Work out the finished part from the listing and answer in its coordinate system (mm). A direction names the side the tool comes from. Give positions to 0.01 mm unless a question says otherwise; leave off trailing zeros. Loops run counter-clockwise (first coordinate to the right, second up) from the corner with the lowest first, then second, coordinate; pieces in that order, holes last.
Autodesk Inventor part; units mm, degrees
ref_plane "YZ Plane" through (0, 0, 0) normal (1, 0, 0) x (0, 1, 0)
ref_plane "XZ Plane" through (0, 0, 0) normal (0, 1, 0) x (-1, 0, 0)
ref_plane "XY Plane" through (0, 0, 0) normal (0, 0, 1) x (1, 0, 0)
sketch "Sketch1" plane through (0, 0, 0) normal (0, 0, 1) x (1, 0, 0)
  circle A0 centre (0, 0) radius 59
  circle A1 centre (90, 0) radius 59
  line L0 (0, 59) -> (90, 59)
  line L1 (90, -59) -> (0, -59)
  dimension "d0" = 118
  dimension "d1" = 118
  dimension "d2" = 90
extrude "Extrusion1" add sketch "Sketch1" along normal blind 5
sketch "Sketch2" plane through (0, 0, 0) normal (0, 0, -1) x (-1, 0, 0)
  arc A0 (0, -59) -> (0, 59) centre (0, 0) ccw
  line L0 (-90, 59) -> (0, 59)
  arc A1 (-90, 59) -> (-90, -59) centre (-90, 0) ccw
  line L1 (0, -59) -> (-90, -59)
  arc A2 (0, -56) -> (0, 56) centre (0, 0) ccw
  line L2 (0, -56) -> (-90, -56)
  arc A3 (-90, 56) -> (-90, -56) centre (-90, 0) ccw
  line L3 (-90, 56) -> (0, 56)
  dimension "d5" = 3
extrude "Extrusion2" cut sketch "Sketch2" against normal blind 4 contours L2 A3 L3 A2
sketch "Sketch3" plane through (0, 0, 5) normal (0, 0, 1) x (1, 0, 0)
  circle A0 centre (90, 0) radius 7.5
  arc A1 (90, -59) -> (90, 59) centre (90, 0) ccw
  circle A2 centre (0, 0) radius 50
  dimension "d8" = 15
  dimension "d9" = 100
extrude "Extrusion3" cut sketch "Sketch3" against normal through all
sketch "Sketch4" plane through (0, 0, 5) normal (0, 0, 1) x (1, 0, 0)
  line L0 (45, 52.5) -> (45, -52.5) construction
  line L1 (90, 59) -> (0, 59) construction
  circle A0 centre (45, 52.5) radius 1.5
  circle A1 centre (45, -52.5) radius 1.5
  point P0 (0, 0)
  point P1 (45, 0)
  point P2 (45, 59)
  dimension "d12" = 105
  dimension "d13" = 3
  dimension "d14" = 3
extrude "Extrusion4" cut sketch "Sketch4" against normal through all
sketch "Sketch5" plane through (0, 0, 4) normal (0, 0, -1) x (-1, 0, 0)
  circle A0 centre (-45, -52.5) radius 1.5
  circle A1 centre (-45, 52.5) radius 1.5
  circle A2 centre (-45, 52.5) radius 6.5
  line L0 (-38.5, 52.5) -> (-38.5, 59)
  line L1 (-51.5, 52.5) -> (-51.5, 59)
  line L2 (-90, 59) -> (0, 59)
  line L3 (-38.5, 59) -> (-51.5, 59)
  line L4 (-51.5, 59) -> (-38.5, 59)
  circle A3 centre (-45, -52.5) radius 6.5
  line L5 (-38.5, -52.5) -> (-38.5, -59)
  line L6 (0, -59) -> (-90, -59)
  line L7 (-38.5, -59) -> (-51.5, -59)
  line L8 (-51.5, -59) -> (-51.5, -52.5)
  point P0 (0, 0)
  dimension "d17" = 13
  dimension "d18" = 13
extrude "Extrusion5" add sketch "Sketch5" along normal blind 4
sketch "Sketch6" plane through (0, 0, 5) normal (0, 0, 1) x (1, 0, 0)
  circle A0 centre (45, -52.5) radius 1.5
  circle A1 centre (45, 52.5) radius 1.5
  circle A2 centre (45, 52.5) radius 1.5
  circle A3 centre (45, 52.5) radius 3
  circle A4 centre (45, -52.5) radius 3
  point P0 (0, 0)
  dimension "d21" = 6
  dimension "d22" = 6
extrude "Extrusion6" cut sketch "Sketch6" against normal blind 3 contours A0 | A1 | A3 | A4
properties part number "HA013" material "ABS Plastic"
Q1. Consider line 1 along Y through (x, z) = (45, 1.2); line 2 along Y through (x, z) = (69.5, 0.95); line 3 along Z through (x, y) = (63, 37.5). Determine where each line is inside the solid, lowest interval first.
Q2. Section A-A on z = 2.9 is taken. Give the vertices of the cut face in (x, y).
Q3. Given pin 1 (1.5 mm diameter, centred on y = -33.5, z = 2, fed in from +X); pin 2 (1 mm diameter, centred on y = -53.5, z = 2, fed in from -X); pin 3 (3.5 mm diameter, centred on x = 45, y = -52.5, fed in from +Z); pin 4 (1.8 mm diameter, centred on x = 45, y = 52.5, fed in from +Z), each flat-ended and moving along its own axis, determine where each tip first touches the part or whether it passes through.
Q4. Section C-C on x = 31 is taken. Give the vertices of the cut face in (y, z), plus the area to 3 significant figures.
Q5. Which of the six approach directions +Z, -Z, +X, -X, +Y, -Y give full straight-line access (tool end or side, diameter ignored) to faces 5 (the face through (44.609, -49.526, 3.521)), 6 (the face through (82.507, 0.33, 4.507)), 7 (the face through (45, 46, 2))?
Q6. Determine the mould class of faces 1 (the face through (148.986, 1.297, 2.465)), 2 (the face through (45, -46, 2)), 3 (the face through (46, 54, 2)), 4 (the face through (-58.986, -1.297, 2.465)) for opening direction X: +X half, -X half, draft (parallel to the pull), parting line (faces both ways), or undercut.
Q7. Section B-B on y = 0 is taken. Give the vertices of the cut face in (x, z), plus the area to 3 significant figures.
Q8. Section D-D on y = -23.5 is taken. Give the vertices of the cut face in (x, z), plus the area to 3 significant figures.
Check result:
1. line 1: y = -59 to -54, -51 to -46, 46 to 51, 54 to 59
1. line 2: y = -59 to -56, 56 to 59
1. line 3: z = 4 to 5
2. outline: (0, -59) - (90, -59) arc R59 ccw to (90, 59) - (0, 59) arc R59 ccw to start; hole (0, -56) - (38.5, -56) - (38.5, -52.5) arc R6.5 cw to (51.5, -52.5) - (51.5, -56) - (90, -56) arc R56 ccw to (90, 56) - (51.5, 56) - (51.5, 52.5) arc R6.5 cw to (38.5, 52.5) - (38.5, 56) - (0, 56) arc R56 ccw to start; hole circle Ø6 at (45, -52.5); hole circle Ø6 at (45, 52.5)
3. pin 1: stops at x = 139.08
3. pin 2: stops at x = -25.92
3. pin 3: stops at z = 2
3. pin 4: passes through
4. outline: (-59, 0) - (-56, 0) - (-56, 4) - (-39.23, 4) - (-39.23, 5) - (-59, 5) - close; (39.23, 4) - (56, 4) - (56, 0) - (59, 0) - (59, 5) - (39.23, 5) - close
4. area: 63.5 mm2
5. face 5: +Z
5. face 6: +Z, -Z
5. face 7: -Z
6. face 1: +X half
6. face 2: undercut
6. face 3: undercut
6. face 4: -X half
7. outline: (-59, 0) - (-56, 0) - (-56, 4) - (-50, 4) - (-50, 5) - (-59, 5) - close; (50, 4) - (82.5, 4) - (82.5, 5) - (50, 5) - close; (97.5, 4) - (146, 4) - (146, 0) - (149, 0) - (149, 5) - (97.5, 5) - close
7. area: 117 mm2
8. outline: (-54.12, 0) - (-50.83, 0) - (-50.83, 4) - (-44.13, 4) - (-44.13, 5) - (-54.12, 5) - close; (44.13, 4) - (140.83, 4) - (140.83, 0) - (144.12, 0) - (144.12, 5) - (44.13, 5) - close
8. area: 136 mm2
